```python
from build123d import *

# Parameters (mm, degrees)
SKETCH1_W           = 113
SKETCH1_H           = 81
BOSS_EXTRUDE1_DEPTH = 1
SKETCH2_W           = 113
SKETCH2_H           = 81
SKETCH2_W_2         = 111
SKETCH2_H_2         = 79
BOSS_EXTRUDE3_DEPTH = 42
CUT_EXTRUDE2_REACH  = 129.508
SKETCH3_W           = 51
SKETCH3_H           = 16
SKETCH4_R           = 1.55
SKETCH4_R_2         = 0.55
BOSS_EXTRUDE4_DEPTH = 1.1
CUT_EXTRUDE3_REACH  = 109.714
SKETCH6_R           = 1.35


with BuildPart() as part:
    # Sketch1 → Boss-Extrude1 (new body)
    with BuildSketch(Plane(origin=(0, 0, 0), x_dir=(1, 0, 0), z_dir=(0, 1, 0))):
        Rectangle(SKETCH1_W, SKETCH1_H)
    extrude(amount=BOSS_EXTRUDE1_DEPTH)

    # Sketch2 → Boss-Extrude3 (add)
    with BuildSketch(Plane(origin=(0, 1, 0), x_dir=(1, 0, 0), z_dir=(0, 1, 0))):
        Rectangle(SKETCH2_W, SKETCH2_H)
        Rectangle(SKETCH2_W_2, SKETCH2_H_2, mode=Mode.SUBTRACT)
    extrude(amount=BOSS_EXTRUDE3_DEPTH)

    # Sketch3 → Cut-Extrude2 (cut, up to next)
    with BuildSketch(Plane(origin=(56.5, 0, 0), x_dir=(0, 0, -1), z_dir=(1, 0, 0)), mode=Mode.PRIVATE) as cut_extrude2_sk1:
        with Locations((-6, 15)):
            Rectangle(SKETCH3_W, SKETCH3_H)
    cut_extrude2_tool1 = extrude(cut_extrude2_sk1.sketch, amount=-CUT_EXTRUDE2_REACH, mode=Mode.PRIVATE) & part.part
    add(cut_extrude2_tool1.solids().sort_by_distance((56.5, 15, 6))[0], mode=Mode.SUBTRACT)

    # Sketch4 → Boss-Extrude4 (add)
    # profile 1 of 2: a face of its own
    with BuildSketch(Plane(origin=(0, 1, 0), x_dir=(1, 0, 0), z_dir=(0, 1, 0))):
        with Locations(Location((52.05, 34.25, 0), (0, 0, 90))):
            Circle(SKETCH4_R)
        with Locations(Location((52.05, 34.25, 0), (0, 0, 270))):
            Circle(SKETCH4_R_2, mode=Mode.SUBTRACT)
    # profile 2 of 2: a face of its own
    with BuildSketch(Plane(origin=(0, 1, 0), x_dir=(1, 0, 0), z_dir=(0, 1, 0))):
        with Locations(Location((-52.05, -35.5, 0), (0, 0, 90))):
            Circle(SKETCH4_R)
        with Locations(Location((-52.05, -35.5, 0), (0, 0, 270))):
            Circle(SKETCH4_R_2, mode=Mode.SUBTRACT)
    extrude(amount=BOSS_EXTRUDE4_DEPTH)

    # Sketch6 → Cut-Extrude3 (cut, up to next)
    with BuildSketch(Plane(origin=(0, 0, -40.5), x_dir=(-1, 0, 0), z_dir=(0, 0, -1)), mode=Mode.PRIVATE) as cut_extrude3_sk1:
        with Locations((-46.35, 24.55)):
            Circle(SKETCH6_R)
    cut_extrude3_tool1 = extrude(cut_extrude3_sk1.sketch, amount=-CUT_EXTRUDE3_REACH, mode=Mode.PRIVATE) & part.part
    # Sketch6 → Cut-Extrude3 (cut, up to next)
    with BuildSketch(Plane(origin=(0, 0, -40.5), x_dir=(-1, 0, 0), z_dir=(0, 0, -1)), mode=Mode.PRIVATE) as cut_extrude3_sk2:
        with Locations((43.95, 19.35)):
            Circle(SKETCH6_R)
    cut_extrude3_tool2 = extrude(cut_extrude3_sk2.sketch, amount=-CUT_EXTRUDE3_REACH, mode=Mode.PRIVATE) & part.part
    add(cut_extrude3_tool1.solids().sort_by_distance((46.35, 24.55, -40.5))[0], mode=Mode.SUBTRACT)
    add(cut_extrude3_tool2.solids().sort_by_distance((-43.95, 19.35, -40.5))[0], mode=Mode.SUBTRACT)


solid = part.part
```
Here's how the part is built. I have some questions about the finished solid (model axes, mm). A direction names the side the tool comes from. Round coordinates to 2 decimals unless told otherwise and drop trailing zeros. Order: outer loops, then holes, each group sorted by start corner. A loop starts at its lowest first (then second) coordinate and runs counter-clockwise, first axis right, second up. Notation, with made-up numbers: (-15.75, 34) -> (-10.75, 34) arc R22 ccw to (-10.75, 69) -> close; hole circle Ø4 at (23.5, 4.25). An arc over 180 degrees is marked (long way). Use a Markdown table: item, result. Add a question column.
(1) Suppose I cut it at A-A, the plane x = 46.35. Please give me the cut outline in (y, z), and give its area (3 significant figures).
(2) I need wall thicknesses on line 1 along Z through (x, y) = (52.05, 1.2); line 2 along Z through (x, y) = (-52.05, 1.8); line 3 along X through (y, z) = (1.45, 35.5). Which ranges of each line are inside material? Lowest first, please.
(3) If we mould it in two halves opening along X, with no side actions, what happens to faces 1 (the face through (-1, 22, -39.5)), 2 (the face through (-56.5, 21, 1)), 3 (the face through (-1, 0, -1))? For each: released by +X, released by -X, zero draft, split by the parting line, or undercut.
(4) Suppose I cut it at D-D, the plane y = 33. Please give me the cut outline in (x, z).
(5) Suppose I cut it at C-C, the plane y = 19.35. Please give me the cut outline in (x, z), and give its area (3 significant figures).
(6) For faces 4 (the face through (45.062, 24.956, -40.007)), 5 (the face through (-1, 21, -40.5)), 6 (the face through (-51, 2.1, 36)), which set-ups out of +Z, -Z, +X, -X, +Y, -Y let a thin tool reach every point of the face, with its end or its side?
(7) Suppose I cut it at B-B, the plane z = 12. Please give me the cut outline in (x, y), and give its area (3 significant figures).
(8) For pin 1 Ø0.5 at (x, z) = (52, -34.5) entering from +Y; pin 2 Ø1.5 at (y, z) = (10.5, -5) entering from +X; pin 3 Ø3.5 at (x, z) = (52, -35) entering from +Y, each with a flat end and sliding along its axis, tell me the tip position at first contact or that it passes through.
Verdict:
| question | item | result |
|---|---|---|
| 1 | outline | (0, -40.5) -> (23.2, -40.5) -> (23.2, -39.5) -> (1, -39.5) -> (1, 39.5) -> (43, 39.5) -> (43, 40.5) -> (0, 40.5) -> close; (25.9, -40.5) -> (43, -40.5) -> (43, -39.5) -> (25.9, -39.5) -> close |
| 1 | area | 162 mm2 |
| 2 | line 1 | -40.5 to -39.5, -35.8 to -34.8, -33.7 to -32.7, 39.5 to 40.5 |
| 2 | line 2 | -40.5 to -39.5, 33.95 to 34.95, 36.05 to 37.05, 39.5 to 40.5 |
| 2 | line 3 | -56.5 to -55.5, -53.6 to -52.6, -51.5 to -50.5, 55.5 to 56.5 |
| 3 | face 1 | undercut |
| 3 | face 2 | released by -X |
| 3 | face 3 | zero draft |
| 4 | outline | (-56.5, -40.5) -> (56.5, -40.5) -> (56.5, 40.5) -> (-56.5, 40.5) -> close; hole (-55.5, -39.5) -> (55.5, -39.5) -> (55.5, 39.5) -> (-55.5, 39.5) -> close |
| 5 | outline | (-56.5, -40.5) -> (-45.3, -40.5) -> (-45.3, -39.5) -> (-55.5, -39.5) -> (-55.5, 39.5) -> (55.5, 39.5) -> (55.5, 31.5) -> (56.5, 31.5) -> (56.5, 40.5) -> (-56.5, 40.5) -> close; (-42.6, -40.5) -> (56.5, -40.5) -> (56.5, -19.5) -> (55.5, -19.5) -> (55.5, -39.5) -> (-42.6, -39.5) -> close |
| 5 | area | 330 mm2 |
| 6 | face 4 | -Z |
| 6 | face 5 | -Z, +X, -X, +Y, -Y |
| 6 | face 6 | +Y |
| 7 | outline | (-56.5, 0) -> (56.5, 0) -> (56.5, 7) -> (55.5, 7) -> (55.5, 1) -> (-55.5, 1) -> (-55.5, 43) -> (-56.5, 43) -> close; (55.5, 23) -> (56.5, 23) -> (56.5, 43) -> (55.5, 43) -> close |
| 7 | area | 181 mm2 |
| 8 | pin 1 | y = 1 |
| 8 | pin 2 | x = -55.5 |
| 8 | pin 3 | y = 2.1 |
